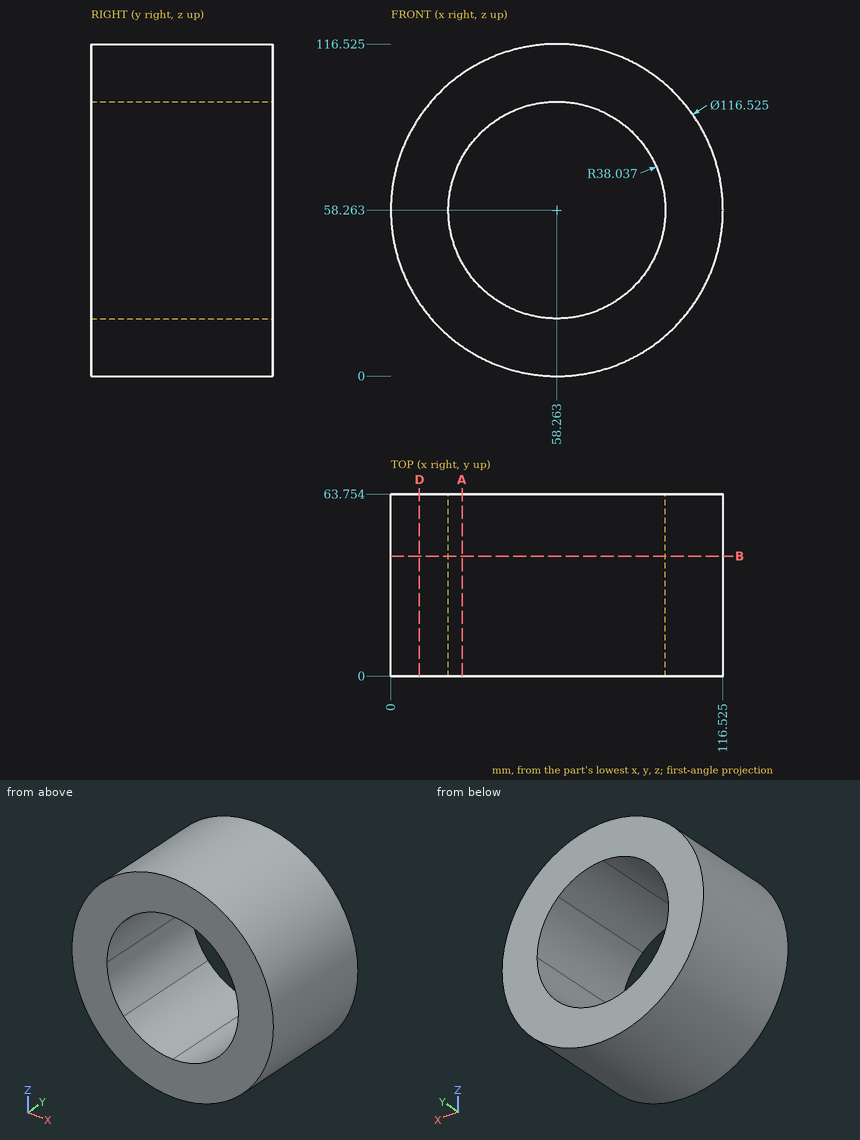
Here's the drawing with two shaded views (mm, measured from the low corner). I have some questions. Give positions to 0.01 mm unless a question says otherwise; leave off trailing zeros. Loops run counter-clockwise (first coordinate to the right, second up) from the corner with the lowest first, then second, coordinate; pieces in that order, holes last. Notation, with made-up numbers: M 35,-12 L 45,-12 A7 cw 45,-7 Z; hole C 50,33.5 d7. An arc over 180 degrees is marked long. Use one line per item in the form item = value. Start each with the question number.
Q1. If we section it at B-B (y = 42): Write out the boundary of the cut face in (x, z) (1 decimal), then the cut area to 3 significant figures.
Q2. If we section it at A-A (x = 25): Write out the boundary of the cut face in (y, z), then the cut area to 3 significant figures.
Q3. If we section it at D-D (x = 10): Write out the boundary of the cut face in (y, z) (1 decimal).
Q4. I need wall thicknesses on line 1 along Z through (x, y) = (57, 18); line 2 along Z through (x, y) = (38, 17) (1 decimal); line 3 along X through (y, z) = (36, 76) (1 decimal). Which ranges of each line are inside material? Lowest first, please.
Q5. Will these pins go through, and if not, where does the flat tip stop? pin 1 Ø2 at (x, y) = (50, 35.5) entering from +Z; pin 2 Ø8 at (y, z) = (42, 14) entering from +X (1 decimal); pin 3 Ø6 at (x, y) = (15.5, 11) entering from +Z.
Taken from the geometry:
q1.outline = C 58.3,58.3 d116.5; hole M 20.2,58.3 A38 ccw 29.8,33 A38 ccw 58.3,20.2 A38 ccw 85.3,31.5 A38 ccw 96.3,58.3 A38 ccw 84.1,86.2 A38 ccw 58.3,96.3 A38 ccw 28.5,82 A38 ccw Z
q1.area = 6,120 mm^2
q2.outline = M 0,10.43 L 63.75,10.43 L 63.75,39.81 L 0,39.81 Z; M 0,76.71 L 63.75,76.71 L 63.75,106.1 L 0,106.1 Z
q2.area = 3,750 mm^2
q3.outline = M 0,25.6 L 63.8,25.6 L 63.8,90.9 L 0,90.9 Z
q4.line_1 = 0.01 to 20.25, 96.28 to 116.51
q4.line_2 = 3.6 to 26.1, 90.5 to 112.9
q4.line_3 = 2.8 to 24.6, 91.9 to 113.8
q5.pin_1 = 116.07
q5.pin_2 = 100.4
q5.pin_3 = 100.85
